Model file for the job. Use its own axes, mm. Give positions to 0.01 mm unless a question says otherwise; leave off trailing zeros. Write each loop counter-clockwise with the first axis right and the second up, starting at its lowest first coordinate (ties: lowest second). Pieces come first, ordered by that corner, then holes.
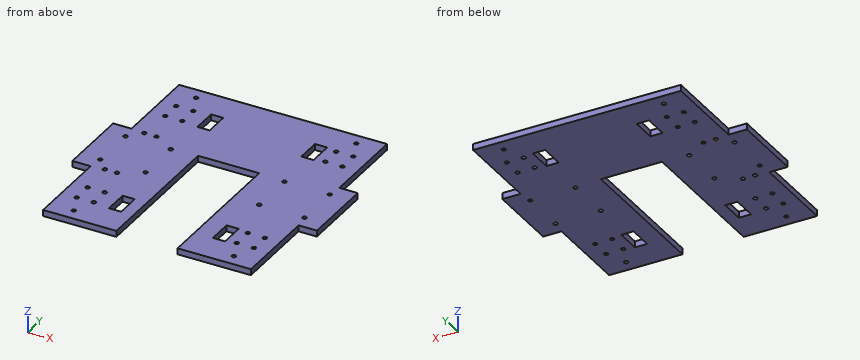
```python
from build123d import *

# Parameters (mm, degrees)
MODEL_R         = 1.65
EXTRUDE_1_DEPTH = 5


with BuildPart() as part:
    # Model → 凸台-拉伸1 (new body)
    with BuildSketch(Plane.XY):
        Polygon((202.712050333, 317.514034213), (372.712050333, 317.514034213), (372.712050333, 247.514034213), (387.712050333, 247.514034213), (387.712050333, 187.514034213), (372.712050333, 187.514034213), (372.712050333, 117.514034213), (312.712050333, 117.514034213), (312.712050333, 237.514034213), (262.712050333, 237.514034213), (262.712050333, 117.514034213), (202.712050333, 117.514034213), (202.712050333, 187.514034213), (187.712050333, 187.514034213), (187.712050333, 247.514034213), (202.712050333, 247.514034213), align=None)
        with Locations((204.212050333, 236.014034213)):
            Circle(MODEL_R, mode=Mode.SUBTRACT)
        with Locations((222.212050333, 127.514034213)):
            Circle(MODEL_R, mode=Mode.SUBTRACT)
        with Locations((353.212050333, 127.514034213)):
            Circle(MODEL_R, mode=Mode.SUBTRACT)
        with Locations((222.212050333, 307.514034213)):
            Circle(MODEL_R, mode=Mode.SUBTRACT)
        with Locations((353.212050333, 307.514034213)):
            Circle(MODEL_R, mode=Mode.SUBTRACT)
        with Locations((241.212050333, 236.014034213)):
            Circle(MODEL_R, mode=Mode.SUBTRACT)
        with Locations((204.212050333, 199.014034213)):
            Circle(MODEL_R, mode=Mode.SUBTRACT)
        with Locations((241.212050333, 199.014034213)):
            Circle(MODEL_R, mode=Mode.SUBTRACT)
        with Locations((371.212050333, 236.014034213)):
            Circle(MODEL_R, mode=Mode.SUBTRACT)
        with Locations((334.212050333, 236.014034213)):
            Circle(MODEL_R, mode=Mode.SUBTRACT)
        with Locations((371.212050333, 199.014034213)):
            Circle(MODEL_R, mode=Mode.SUBTRACT)
        with Locations((334.212050333, 199.014034213)):
            Circle(MODEL_R, mode=Mode.SUBTRACT)
        with Locations((215.212050333, 290.514034213)):
            Circle(MODEL_R, mode=Mode.SUBTRACT)
        with Locations((229.212050333, 290.514034213)):
            Circle(MODEL_R, mode=Mode.SUBTRACT)
        with Locations((215.212050333, 274.514034213)):
            Circle(MODEL_R, mode=Mode.SUBTRACT)
        with Locations((229.212050333, 274.514034213)):
            Circle(MODEL_R, mode=Mode.SUBTRACT)
        with Locations((215.212050333, 144.514034213)):
            Circle(MODEL_R, mode=Mode.SUBTRACT)
        with Locations((215.212050333, 160.514034213)):
            Circle(MODEL_R, mode=Mode.SUBTRACT)
        with Locations((360.212050333, 290.514034213)):
            Circle(MODEL_R, mode=Mode.SUBTRACT)
        with Locations((346.212050333, 290.514034213)):
            Circle(MODEL_R, mode=Mode.SUBTRACT)
        with Locations((360.212050333, 274.514034213)):
            Circle(MODEL_R, mode=Mode.SUBTRACT)
        with Locations((346.212050333, 274.514034213)):
            Circle(MODEL_R, mode=Mode.SUBTRACT)
        with Locations((360.212050333, 144.514034213)):
            Circle(MODEL_R, mode=Mode.SUBTRACT)
        with Locations((360.212050333, 160.514034213)):
            Circle(MODEL_R, mode=Mode.SUBTRACT)
        with Locations((229.212050333, 144.514034213)):
            Circle(MODEL_R, mode=Mode.SUBTRACT)
        with Locations((229.212050333, 160.514034213)):
            Circle(MODEL_R, mode=Mode.SUBTRACT)
        with Locations((346.212050333, 144.514034213)):
            Circle(MODEL_R, mode=Mode.SUBTRACT)
        with Locations((346.212050333, 160.514034213)):
            Circle(MODEL_R, mode=Mode.SUBTRACT)
        with Locations((223.712050333, 246.514034213)):
            Circle(MODEL_R, mode=Mode.SUBTRACT)
        with Locations((213.712050333, 246.442167925)):
            Circle(MODEL_R, mode=Mode.SUBTRACT)
        with Locations((223.712050333, 188.514034213)):
            Circle(MODEL_R, mode=Mode.SUBTRACT)
        with Locations((213.712050333, 188.585900501)):
            Circle(MODEL_R, mode=Mode.SUBTRACT)
        Polygon((252.712050333, 142.514034213), (247.712050333, 142.514034213), (242.712050333, 142.514034213), (242.712050333, 162.514034213), (252.712050333, 162.514034213), align=None, mode=Mode.SUBTRACT)
        Polygon((327.712050333, 142.514034213), (332.712050333, 142.514034213), (337.712050333, 142.514034213), (337.712050333, 162.514034213), (327.712050333, 162.514034213), align=None, mode=Mode.SUBTRACT)
        Polygon((252.712050333, 292.514034213), (247.712050333, 292.514034213), (242.712050333, 292.514034213), (242.712050333, 272.514034213), (252.712050333, 272.514034213), align=None, mode=Mode.SUBTRACT)
        Polygon((327.712050333, 292.514034213), (332.712050333, 292.514034213), (337.712050333, 292.514034213), (337.712050333, 272.514034213), (327.712050333, 272.514034213), align=None, mode=Mode.SUBTRACT)
    extrude(amount=EXTRUDE_1_DEPTH)


solid = part.part
```
1. Probe probe 1 along X at (y, z) = (156, 3); probe 2 along X at (y, z) = (134, 3.1); probe 3 along X at (y, z) = (223.5, 4.4). List the from-to ranges inside material, lowest first.
Calculated:
probe 1: x = 202.71 to 242.71, 252.71 to 262.71, 312.71 to 327.71, 337.71 to 372.71
probe 2: x = 202.71 to 262.71, 312.71 to 372.71
probe 3: x = 187.71 to 262.71, 312.71 to 387.71
2. Pin check, flat tips, straight feed: P1, Ø4.5, axis at x = 215.21, y = 144.51, coming from the -Z side; P2, Ø1.5, axis at y = 278.5, z = 2, coming from the +X side; P3, Ø3, axis at y = 251.5, z = 4, coming from the -X side. Stop position of each tip, or through.
Calculated:
P1: stops at z = 0
P2: stops at x = 372.71
P3: stops at x = 202.71
3. Slice it at A-A, the plane y = 218.5. Write the cut outline in (x, z), and give its area (3 significant figures).
Calculated:
outline: (187.71, 0) - (262.71, 0) - (262.71, 5) - (187.71, 5) - close; (312.71, 0) - (387.71, 0) - (387.71, 5) - (312.71, 5) - close
area: 750 mm2
4. Slice it at C-C, the plane y = 300.5. Write the cut outline in (x, z).
Calculated:
outline: (202.71, 0) - (372.71, 0) - (372.71, 5) - (202.71, 5) - close
5. Slice it at D-D, the plane z = 3.8. State how many separate pieces and enclosed holes the cut face has, and give its area (3 significant figures).
Calculated:
separate pieces: 1
enclosed holes: 36
area: 28,700 mm2
6. Slice it at B-B, the plane x = 278.5. Write the cut outline in (y, z).
Calculated:
outline: (237.51, 0) - (317.51, 0) - (317.51, 5) - (237.51, 5) - close
